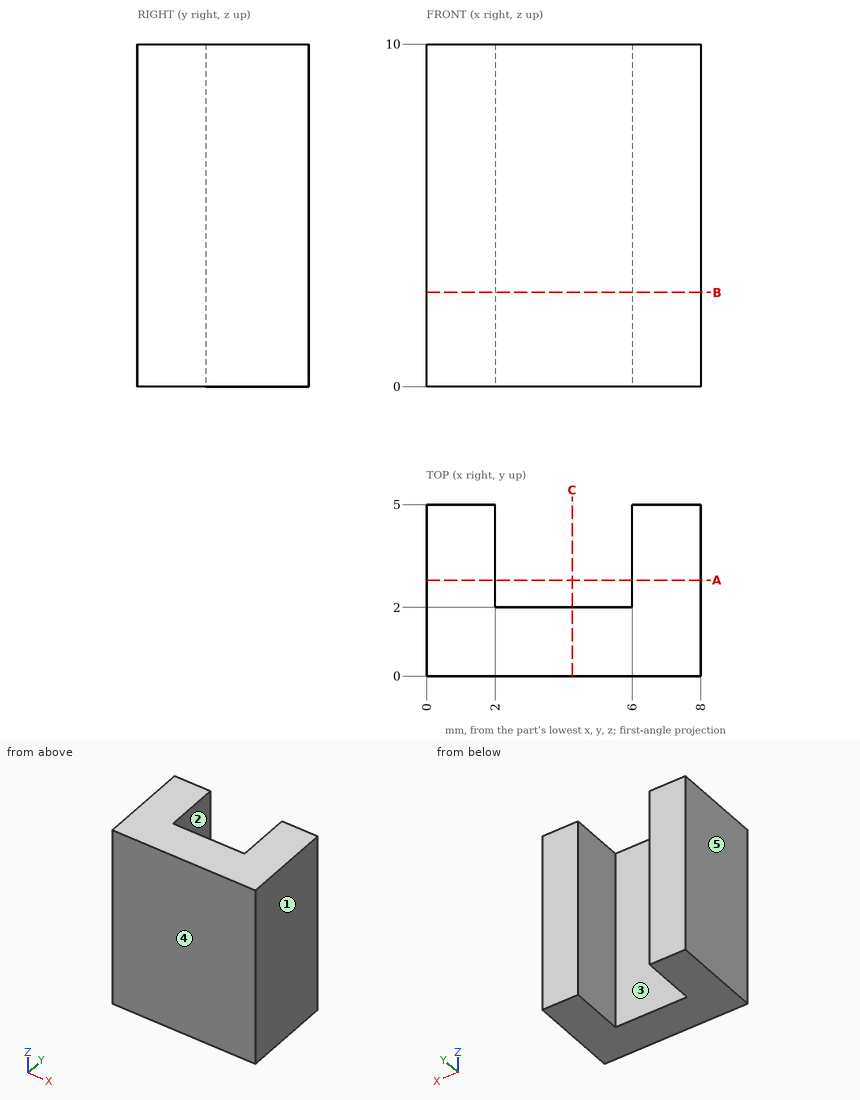
Study the drawing (mm; zero at the part's minimum x, y, z) and answer. A direction names the side the tool comes from. Give positions to 0.01 mm unless a question says otherwise; leave off trailing zeros. Order: outer loops, then holes, each group sorted by start corner. A loop starts at its lowest first (then second) coordinate and runs counter-clockwise, first axis right, second up. Notation, with made-up numbers: M 5,75.5 L 27,75.5 A14 cw 27,98.5 Z; hole C 60.5,-14 d11. An arc over 180 degrees is marked long. Put each result on its own line as item: value. Start each with the question number.
Item 1: The part is cut by section B-B, the plane z = 2.75. Determine the outline of the cut face in (x, y), and give its area (3 significant figures).
Item 2: The part is cut by section A-A, the plane y = 2.8. Determine the outline of the cut face in (x, z), and give its area (3 significant figures).
Item 3: Find the intervals of material crossed by line 1 along X through (y, z) = (4.75, 8.75); line 2 along Y through (x, z) = (3.25, 2.25), in increasing order.
Item 4: The part is cut by section C-C, the plane x = 4.25. Determine the outline of the cut face in (y, z).
Item 5: For a pull along X with two mould halves and no side action, classify the marked faces 3, 4 and 5 as +X half, -X half, draft (parallel to the pull), parting line (faces both ways), or undercut.
Item 6: Which of the six approach directions +Z, -Z, +X, -X, +Y, -Y give full straight-line access (tool end or side, diameter ignored) to the marked faces 1 and 2?
Item 7: A flat-ended cylindrical pin translates along its axis: P1, Ø4.5, axis at x = 4.5, z = 3.5, coming from the +Y side. Find the tip coordinate at first contact, or state that the pin passes through.
Answer key:
1. outline: M 0,0 L 8,0 L 8,5 L 6,5 L 6,2 L 2,2 L 2,5 L 0,5 Z
1. area: 28.0 mm²
2. outline: M 0,0 L 2,0 L 2,10 L 0,10 Z; M 6,0 L 8,0 L 8,10 L 6,10 Z
2. area: 40.0 mm²
3. line 1: x = 0 to 2, 6 to 8
3. line 2: y = 0 to 2
4. outline: M 0,0 L 2,0 L 2,10 L 0,10 Z
5. face 3: undercut
5. face 4: draft
5. face 5: -X half
6. face 1: +Z, -Z, +X, +Y, -Y
6. face 2: +Z, -Z, +Y
7. P1: stops at y = 5
